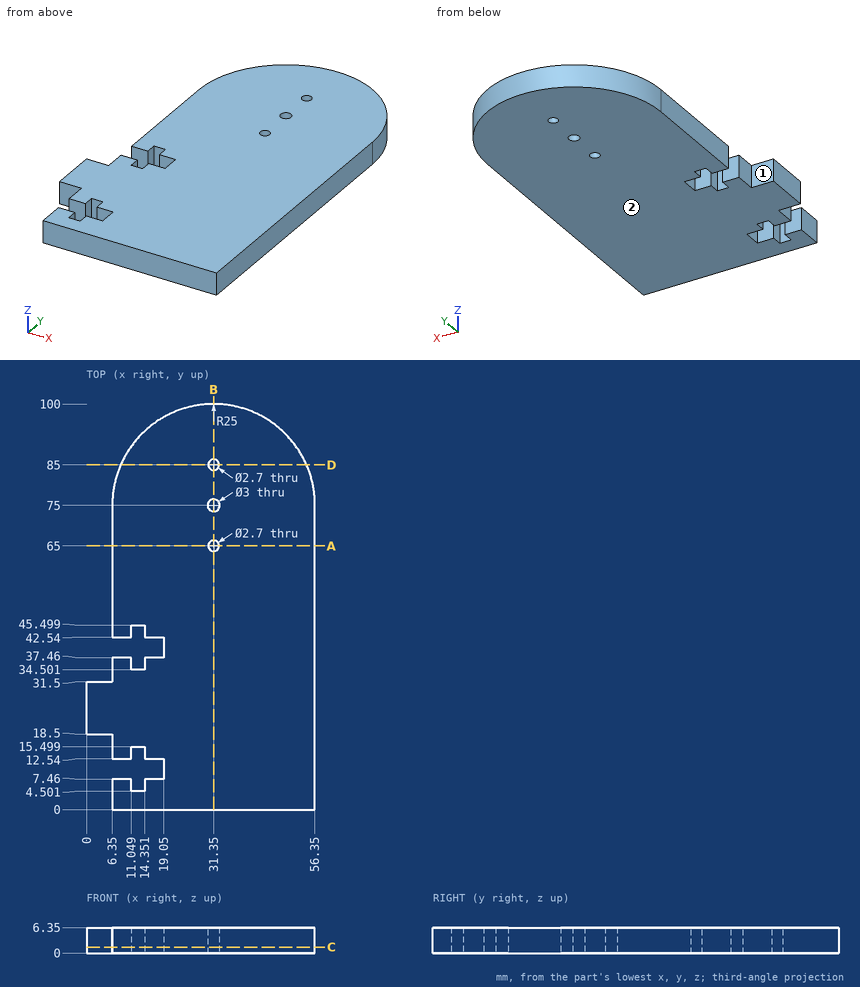
Here's the drawing with two shaded views (mm, measured from the low corner). I have some questions. A direction names the side the tool comes from. Round coordinates to 2 decimals unless told otherwise and drop trailing zeros. Loops run counter-clockwise (first coordinate to the right, second up) from the corner with the lowest first, then second, coordinate; pieces in that order, holes last. Notation, with made-up numbers: (31, 73.5) - (35, 73.5) arc R19 ccw to (35, 84.5) - close; hole circle Ø5 at (40.5, -5). An arc over 180 degrees is marked (long way). Write item = value, one per line.
1) Imagine slicing it at B-B (x = 31.35). Please give me the cut outline in (y, z), and give its area (3 significant figures).
Computed:
outline = (0, 0) - (63.65, 0) - (63.65, 6.35) - (0, 6.35) - close; (66.35, 0) - (73.5, 0) - (73.5, 6.35) - (66.35, 6.35) - close; (76.5, 0) - (83.65, 0) - (83.65, 6.35) - (76.5, 6.35) - close; (86.35, 0) - (100, 0) - (100, 6.35) - (86.35, 6.35) - close
area = 582 mm2
2) I need wall thicknesses on line 1 along Y through (x, z) = (31.35, 4.5); line 2 along X through (y, z) = (65, 2.5); line 3 along X through (y, z) = (12.5, 2.75). Which ranges of each line are inside material? Lowest first, please. Write a range as from..to.
Computed:
line_1 = 0..63.65, 66.35..73.5, 76.5..83.65, 86.35..100
line_2 = 6.35..30, 32.7..56.35
line_3 = 19.05..56.35
3) On a 3-axis mill with a long thin cutter (end or side, diameter ignored), from which of +Z, -Z, +X, -X, +Y, -Y can I reach the whole of each face in a straight line? I mean the marked faces 1 and 2. Say none if no direction works.
Computed:
face_1 = +Z, -Z, -X, +Y
face_2 = -Z, +X, -X, +Y, -Y
4) Imagine slicing it at A-A (y = 65). Please give me the cut outline in (x, z), and give its area (3 significant figures).
Computed:
outline = (6.35, 0) - (30, 0) - (30, 6.35) - (6.35, 6.35) - close; (32.7, 0) - (56.35, 0) - (56.35, 6.35) - (32.7, 6.35) - close
area = 300 mm2
5) Imagine slicing it at D-D (y = 85). Please give me the cut outline in (x, z), and give its area (3 significant figures).
Computed:
outline = (8.44, 0) - (30, 0) - (30, 6.35) - (8.44, 6.35) - close; (32.7, 0) - (54.26, 0) - (54.26, 6.35) - (32.7, 6.35) - close
area = 274 mm2
6) I'm going to push flat-ended pins straight in: P1, Ø2.5, axis at x = 31.35, y = 65, coming from the +Z side; P2, Ø2.5, axis at x = 17, z = 3, coming from the +Y side; P3, Ø0.9, axis at y = 44, z = 2, coming from the -X side; P4, Ø12, axis at x = 28, y = 65.5, coming from the -Z side. Where does each tip first touch, or does it pass through?
Computed:
P1 = through
P2 = 96.29
P3 = 6.35
P4 = 0
7) Imagine slicing it at C-C (z = 1.5). Give the number of separate pieces and of enclosed holes in the cut face, and give its area (3 significant figures).
Computed:
separate_pieces = 1
enclosed_holes = 3
area = 4,630 mm2
